Could you check a few things on this model? Use its own coordinates, in mm. A direction names the side the tool comes from. Give positions to 0.01 mm unless a question says otherwise; leave off trailing zeros. Write each loop counter-clockwise with the first axis right and the second up, starting at its lowest first coordinate (ties: lowest second). Pieces come first, ordered by that corner, then holes. Notation, with made-up numbers: M 29.25,21 L 83.25,21 A15 ccw 83.25,49 Z; hole C -10,-19 d5. An arc over 180 degrees is marked long. One line per item, written item: value.
```python
from build123d import *

# Parameters (mm, degrees)
SKETCH1_W           = 12
SKETCH1_H           = 20
SKETCH1_R           = 1.5
BOSS_EXTRUDE1_DEPTH = 3
BOSS_EXTRUDE2_DEPTH = 1
FILLET1_R           = 0.25
BOSS_EXTRUDE3_START = 3
SKETCH4_R           = 1.5
BOSS_EXTRUDE3_DEPTH = 3
FILLET2_R           = 1


with BuildPart() as part:
    # Sketch1 → Boss-Extrude1 (new body)
    with BuildSketch(Plane.XY):
        Rectangle(SKETCH1_W, SKETCH1_H)
        with Locations((0, 5)):
            Circle(SKETCH1_R, mode=Mode.SUBTRACT)
        with Locations((0, -5)):
            Circle(SKETCH1_R, mode=Mode.SUBTRACT)
    extrude(amount=BOSS_EXTRUDE1_DEPTH)

    # Sketch3 → Boss-Extrude2 (add)
    with BuildSketch(Plane(origin=(0, 0, 0), x_dir=(-1, 0, 0), z_dir=(0, 0, -1))):
        with BuildLine():
            Line((-2.5, -10), (2.5, -10))
            Line((2.5, -10), (2.5, -7.449489743))
            ThreePointArc((2.5, -7.449489743), (0, -8.5), (-2.5, -7.449489743))
            Line((-2.5, -7.449489743), (-2.5, -10))
        make_face()
        with BuildLine():
            Line((-2.5, 10), (2.5, 10))
            Line((2.5, 10), (2.5, 7.449489743))
            ThreePointArc((2.5, 7.449489743), (0, 8.5), (-2.5, 7.449489743))
            Line((-2.5, 7.449489743), (-2.5, 10))
        make_face()
        with BuildLine():
            Line((2.5, -2.550510257), (2.5, 2.550510257))
            ThreePointArc((2.5, 2.550510257), (0, 1.5), (-2.5, 2.550510257))
            Line((-2.5, 2.550510257), (-2.5, -2.550510257))
            ThreePointArc((-2.5, -2.550510257), (0, -1.5), (2.5, -2.550510257))
        make_face()
    extrude(amount=BOSS_EXTRUDE2_DEPTH)

    # Fillet1
    fillet1_edges = [part.edges().sort_by_distance(p)[0] for p in [
        (2.5, -7.449489743, -0.5),
        (-2.5, -7.449489743, -0.5),
        (-2.5, 7.449489743, -0.5),
        (2.5, 7.449489743, -0.5),
        (-2.5, 2.550510257, -0.5),
        (2.5, 2.550510257, -0.5),
        (2.5, -2.550510257, -0.5),
        (-2.5, -2.550510257, -0.5),
    ]]
    fillet(fillet1_edges, radius=FILLET1_R)

    # Sketch4 → Boss-Extrude3 (add)
    with BuildSketch(Plane(origin=(0, 0, 0), x_dir=(0, 0, -1), z_dir=(1, 0, 0)).offset(BOSS_EXTRUDE3_START)):
        with BuildLine():
            Line((-3, 10), (-9.896551724, 2.75862069))
            ThreePointArc((-9.896551724, 2.75862069), (-11, 0), (-9.896551724, -2.75862069))
            Line((-9.896551724, -2.75862069), (-3, -10))
            Line((-3, -10), (-3, 10))
        make_face()
        with Locations((-7, 0)):
            Circle(SKETCH4_R, mode=Mode.SUBTRACT)
    boss_extrude3 = extrude(amount=BOSS_EXTRUDE3_DEPTH)

    # Mirror2: Boss-Extrude3 across plane
    add(boss_extrude3.mirror(Plane(origin=(0, 0, 0), x_dir=(0, 0, 1), z_dir=(1, 0, 0))))

    # Fillet2
    fillet2_edges = [part.edges().sort_by_distance(p)[0] for p in [
        (6, -10, 1.5),
        (-6, -10, 1.5),
        (-6, 10, 1.5),
        (6, 10, 1.5),
    ]]
    fillet(fillet2_edges, radius=FILLET2_R)


solid = part.part
```
1) Please list where these lines run through material, in increasing order: L1, parallel to Y at x = 0, z = 1.75; L2, parallel to X at y = 1, z = 3.25; L3, parallel to Y at x = 1.25, z = -0.25. Write a range as from..to.
Outcome:
L1: y = -10..-6.5, -3.5..3.5, 6.5..10
L2: x = -6..-3, 3..6
L3: y = -10..-8.27, -1.73..1.73, 8.27..10
2) I'm going to push flat-ended pins straight in: pin 1 (2 mm diameter, centred on x = 1.5, y = 1, fed in from +Z); pin 2 (0.5 mm diameter, centred on y = 9, z = -0.5, fed in from +X); pin 3 (0.5 mm diameter, centred on y = 9.5, z = -0.5, fed in from -X). Where does each tip first touch, or does it pass through?
Outcome:
pin 1: stops at z = 3
pin 2: stops at x = 2.5
pin 3: stops at x = -2.5
3) If we section it at C-C, the plane y = 4.5: Write out the boundary of the cut face in (x, z).
Outcome:
outline: M -6,0 L -1.41,0 L -1.41,3 L -3,3 L -3,8.24 L -6,8.24 Z; M 1.41,0 L 6,0 L 6,8.24 L 3,8.24 L 3,3 L 1.41,3 Z
4) If we section it at B-B, the plane x = -4: Write out the boundary of the cut face in (y, z), then the cut area to 3 significant figures.
Outcome:
outline: M -10,0 L 10,0 L 10,3 L 2.76,9.9 A4 ccw -2.76,9.9 L -10,3 Z; hole C 0,7 d3
area: 145 mm^2
5) If we section it at D-D, the plane y = 0: Write out the boundary of the cut face in (x, z), then the cut area to 3 significant figures.
Outcome:
outline: M -6,0 L -2.5,0 L -2.5,-1 L 2.5,-1 L 2.5,0 L 6,0 L 6,5.5 L 3,5.5 L 3,3 L -3,3 L -3,5.5 L -6,5.5 Z; M -6,8.5 L -3,8.5 L -3,11 L -6,11 Z; M 3,8.5 L 6,8.5 L 6,11 L 3,11 Z
area: 71.0 mm^2
6) We'd pull the mould along Y, two halves only. Please class faces 5 (the face through (0, -1.5, -0.5)), 6 (the face through (0, 10, 1)), 7 (the face through (-2.5, -9, -0.5)): pulls with the +Y half, pulls with the -Y half, needs draft (parallel to the pull), parting line crosses it, or undercut.
Outcome:
face 5: undercut
face 6: pulls with the +Y half
face 7: needs draft
7) If we section it at A-A, the plane z = 7: Write out the boundary of the cut face in (x, y).
Outcome:
outline: M -6,-5.8 L -3,-5.8 L -3,-1.5 L -6,-1.5 Z; M -6,1.5 L -3,1.5 L -3,5.8 L -6,5.8 Z; M 3,-5.8 L 6,-5.8 L 6,-1.5 L 3,-1.5 Z; M 3,1.5 L 6,1.5 L 6,5.8 L 3,5.8 Z
8) On a 3-axis mill with a long thin cutter (end or side, diameter ignored), from which of +Z, -Z, +X, -X, +Y, -Y can I reach the whole of each face in a straight line? I mean faces 1 (the face through (-2.5, 9, -0.5)), 2 (the face through (0, 1.5, -0.5)), 3 (the face through (-3, 0, 5)), 4 (the face through (2.5, 9, -0.5)). Say none if no direction works.
Outcome:
face 1: -Z, -X, +Y, -Y
face 2: -Z
face 3: +Z, +Y, -Y
face 4: -Z, +X, +Y, -Y
